Job drawing, mm, ordinate dimensions from the low corner. One solid piece. Round coordinates to 2 decimals unless told otherwise and drop trailing zeros. Write each loop counter-clockwise with the first axis right and the second up, starting at its lowest first coordinate (ties: lowest second). Pieces come first, ordered by that corner, then holes.
1) Saw through at B-B on x = 36.5. Write the cut outline in (y, z).
2) Saw through at A-A on y = 1.8. Write the cut outline in (x, z).
3) Drill centre lines: L1, parallel to X at y = 3.25, z = 13.5; L2, parallel to Z at x = 7, y = 0.55; L3, parallel to X at y = 1.45, z = 33. Where is each one in solid material? Low to high.
4) Saw through at C-C on z = 30. Write the cut outline in (x, y).
5) Flat gauge pins, fed straight in: pin 1 (1.5 mm diameter, centred on x = 3.5, y = 3, fed in from -Z); pin 2 (8 mm diameter, centred on x = 55, z = 16, fed in from -Y); pin 3 (3 mm diameter, centred on x = 29, y = 3.5, fed in from -Z); pin 4 (1.5 mm diameter, centred on y = 3, z = 51.5, fed in from -X). Where does each tip first touch, or does it go through?
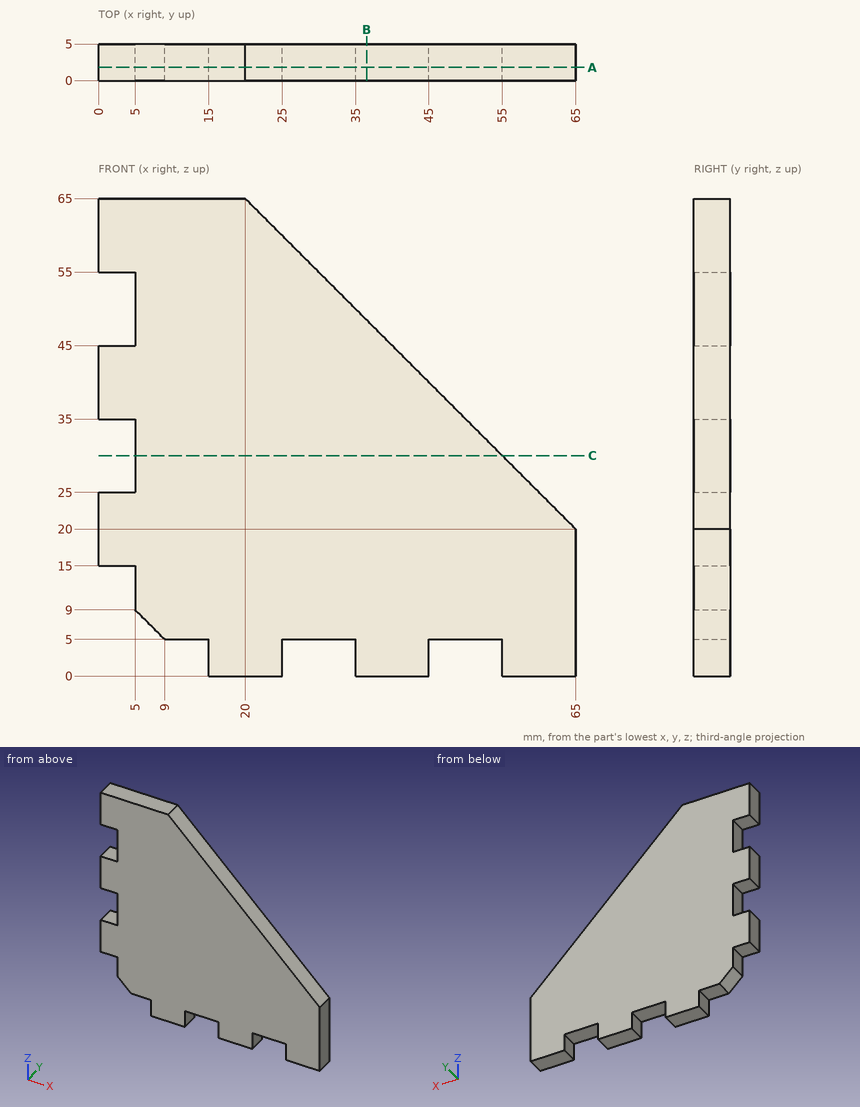
Completed:
1. outline: (0, 0) - (5, 0) - (5, 48.5) - (0, 48.5) - close
2. outline: (0, 15) - (5, 15) - (5, 9) - (9, 5) - (15, 5) - (15, 0) - (25, 0) - (25, 5) - (35, 5) - (35, 0) - (45, 0) - (45, 5) - (55, 5) - (55, 0) - (65, 0) - (65, 20) - (20, 65) - (0, 65) - (0, 55) - (5, 55) - (5, 45) - (0, 45) - (0, 35) - (5, 35) - (5, 25) - (0, 25) - close
3. L1: x = 5 to 65
3. L2: z = 7 to 65
3. L3: x = 5 to 52
4. outline: (5, 0) - (55, 0) - (55, 5) - (5, 5) - close
5. pin 1: stops at z = 15
5. pin 2: stops at y = 0
5. pin 3: stops at z = 5
5. pin 4: stops at x = 5
